CAD build for the part. Positions are in the model's coordinates, mm. A direction names the side the tool comes from. Give positions to 0.01 mm unless a question says otherwise; leave off trailing zeros. Order: outer loops, then holes, each group sorted by start corner. A loop starts at its lowest first (then second) coordinate and runs counter-clockwise, first axis right, second up.
from build123d import *

# Parameters (mm, degrees)
SKETCH1_R           = 1.5
BOSS_EXTRUDE1_DEPTH = 6
SKETCH2_R           = 5.75
SKETCH2_R_2         = 3.1
BOSS_EXTRUDE2_DEPTH = 12
SKETCH3_R           = 1.5
CUT_EXTRUDE1_DEPTH  = 6


with BuildPart() as part:
    # Sketch1 → Boss-Extrude1 (new body)
    with BuildSketch(Plane(origin=(0, 0, 0), x_dir=(1, 0, 0), z_dir=(0, 1, 0))):
        Polygon((6.92820323, 0), (3.464101615, 6), (-3.464101615, 6), (-6.92820323, 0), (-3.464101615, -6), (3.464101615, -6), align=None)
        with Locations(Location((0, 0, 0), (0, 0, 270))):
            Circle(SKETCH1_R, mode=Mode.SUBTRACT)
    extrude(amount=BOSS_EXTRUDE1_DEPTH)

    # Sketch2 → Boss-Extrude2 (add)
    with BuildSketch(Plane(origin=(0, 6, 0), x_dir=(1, 0, 0), z_dir=(0, 1, 0))):
        with Locations(Location((0, 0, 0), (0, 0, 270))):
            Circle(SKETCH2_R)
        with Locations(Location((0, 0, 0), (0, 0, 270))):
            Circle(SKETCH2_R_2, mode=Mode.SUBTRACT)
    extrude(amount=BOSS_EXTRUDE2_DEPTH)

    # Sketch3 → Cut-Extrude1 (cut, symmetric)
    with BuildSketch(Plane(origin=(0, 0, 0), x_dir=(0, 0, -1), z_dir=(1, 0, 0))):
        with Locations((0, 13)):
            Circle(SKETCH3_R)
    extrude(amount=CUT_EXTRUDE1_DEPTH, both=True, mode=Mode.SUBTRACT)


solid = part.part
1. Saw through at D-D on x = 4.5. Give the cut face in (y, z), plus the area to 3 significant figures.
2. Saw through at B-B on x = 0. Give the cut face in (y, z), plus the area to 3 significant figures.
3. Pin check, flat tips, straight feed: P1, Ø5, axis at y = 13, z = 0, coming from the -X side; P2, Ø1.8, axis at x = 0, z = 0, coming from the +Y side; P3, Ø2, axis at x = 2.5, y = 8, coming from the +Z side; P4, Ø1.5, axis at x = -0.5, y = 12, coming from the +Z side. Stop position of each tip, or through.
4. Mould opens along Z. For faces 1 (the cylindrical face through (-5.101, 11.916, 2.653)), 2 (the flat face through (-5.172, 2.958, -3.042)), 3 (the cylindrical face through (-4.213, 12.425, -1.386)) say: released by +Z, released by -Z, zero draft, split by the parting line, or undercut.
5. Wall check: line 1 (Y direction, x = -3.8, z = 0); line 2 (Y direction, x = -2.75, z = -0.75); line 3 (Z direction, x = 1, y = 14). Give the ranges that are in metal, low to high.
6. 3-axis set-ups, long thin cutter, end or side, ignore diameter. For faces 4 (the cylindrical face through (2.61, 11.92, 1.67)), 5 (the flat face through (0, 3, -6)): which of +Z, -Z, +X, -X, +Y, -Y reach the whole face in a straight line?
7. Saw through at C-C on y = 13. Give the cut face in (x, z), plus the area to 3 significant figures.
8. Saw through at A-A on y = 3.25. Give the cut face in (x, z).
Reported:
1. outline: (0, -4.21) - (6, -4.21) - (6, -3.58) - (18, -3.58) - (18, 3.58) - (6, 3.58) - (6, 4.21) - (0, 4.21) - close; hole circle Ø3 at (13, 0)
1. area: 129 mm2
2. outline: (0, -6) - (6, -6) - (6, -5.75) - (18, -5.75) - (18, -3.1) - (6, -3.1) - (6, -1.5) - (0, -1.5) - close; (0, 1.5) - (6, 1.5) - (6, 3.1) - (18, 3.1) - (18, 5.75) - (6, 5.75) - (6, 6) - (0, 6) - close
2. area: 118 mm2
3. P1: stops at x = -5.75
3. P2: passes through
3. P3: stops at z = 5.55
3. P4: stops at z = 5.75
4. face 1: split by the parting line
4. face 2: released by -Z
4. face 3: undercut
5. line 1: y = 0 to 11.5, 14.5 to 18
5. line 2: y = 0 to 6
5. line 3: z = -5.66 to -2.93, 2.93 to 5.66
6. face 4: +Y
6. face 5: -Z, +X, -X, +Y, -Y
7. outline: (-5.55, -1.5) arc R5.75 ccw to (5.55, -1.5) - (2.71, -1.5) arc R3.1 cw to (-2.71, -1.5) - close; (-5.55, 1.5) - (-2.71, 1.5) arc R3.1 cw to (2.71, 1.5) - (5.55, 1.5) arc R5.75 ccw to start
7. area: 57.4 mm2
8. outline: (-6.93, 0) - (-3.46, -6) - (3.46, -6) - (6.93, 0) - (3.46, 6) - (-3.46, 6) - close; hole circle Ø3 at (0, 0)
